from build123d import *

# Parameters (mm, degrees)
SKETCH1_R                   = 79.375
BOSS_EXTRUDE1_DEPTH         = 3.175
TAP_DRILL_FOR_M5X0_8_TAP1_D = 4.2
TAP_DRILL_FOR_M7X1_0_TAP1_D = 6
TAP_DRILL_FOR_M4X0_7_TAP1_D = 3.3


with BuildPart() as part:
    # Sketch1 → Boss-Extrude1 (new, symmetric)
    with BuildSketch(Plane(origin=(0, 0, 0), x_dir=(1, 0, 0), z_dir=(0, 1, 0))):
        with Locations(Location((0, 0, 0), (0, 0, 270))):
            Circle(SKETCH1_R)
    extrude(amount=BOSS_EXTRUDE1_DEPTH, both=True)

    # Tap Drill for M5x0.8 Tap1 (through all)
    with Locations(Plane(origin=(0, 3.175, 0), x_dir=(1, 0, 0), z_dir=(0, 1, 0))):
        with Locations((-27.3188086, 31.571183672), (4.4311914, 31.571183672), (-15.875, -19.245910728), (15.875, -19.245910728)):
            Hole(TAP_DRILL_FOR_M5X0_8_TAP1_D / 2)

    # Tap Drill for M7x1.0 Tap1 (through all)
    with Locations(Plane(origin=(0, 3.175, 0), x_dir=(1, 0, 0), z_dir=(0, 1, 0))):
        with Locations((-44.245, 9.941583672), (-44.245, -15.058416328), (44.245, 9.941583672), (44.245, -15.058416328)):
            Hole(TAP_DRILL_FOR_M7X1_0_TAP1_D / 2)

    # Tap Drill for M4x0.7 Tap1 (through all)
    with Locations(Plane(origin=(0, 3.175, 0), x_dir=(1, 0, 0), z_dir=(0, 1, 0))):
        with Locations((-26.155, -44.384416328), (26.155, -44.384416328)):
            Hole(TAP_DRILL_FOR_M4X0_7_TAP1_D / 2)


solid = part.part
Could you check a few things on this model? Use its own coordinates, in mm. Give positions to 0.01 mm unless a question says otherwise; leave off trailing zeros. Loops run counter-clockwise (first coordinate to the right, second up) from the corner with the lowest first, then second, coordinate; pieces in that order, holes last. Notation, with made-up numbers: M -17,56.5 L 38,56.5 A20 cw 38,94.5 Z; hole C 88,-19.5 d4. An arc over 180 degrees is marked long. Answer as a JSON object with one key per item and string values.
Q1. For P1, Ø1.5, axis at x = 60.5, y = 0.5, coming from the +Z side; P2, Ø2, axis at y = -2, z = -32.5, coming from the +X side; P3, Ø1, axis at x = -23, y = -1, coming from the -Z side, each with a flat end and sliding along its axis, tell me the tip position at first contact or that it passes through.
Values found:
{"P1": "stops at z = 52.25", "P2": "stops at x = 72.86", "P3": "stops at z = -76.12"}
Q2. Suppose I cut it at A-A, the plane y = -0.25. State how many separate pieces and enclosed holes the cut face has, plus the area to 3 significant figures.
Values found:
{"separate pieces": "1", "enclosed holes": "10", "area": "19,600 mm²"}
Q3. If we mould it in two halves opening along Z, with no side actions, what happens to faces 1 (the cylindrical face through (-15.42, -0.044, 21.296)), 2 (the flat face through (1, 3.175, -1)), 3 (the cylindrical face through (23.84, 0.04, 75.71))? For each: pulls with the +Z half, pulls with the -Z half, needs draft (parallel to the pull), parting line crosses it, or undercut.
Values found:
{"face 1": "undercut", "face 2": "needs draft", "face 3": "parting line crosses it"}
Q4. Suppose I cut it at B-B, the plane z = 30. List the corners of the cut face in (x, y) for me (3 decimals).
Values found:
{"outline": "M -73.487,-3.175 L 73.487,-3.175 L 73.487,3.175 L -73.487,3.175 Z"}
Q5. If I drill on probe 1 along X at (y, z) = (-2.5, 21); probe 2 along X at (y, z) = (0.25, -33.5); probe 3 along X at (y, z) = (2.5, 17.5), over which ranges is the centre line in solid material (lowest first)? Write a range as [from, to].
Values found:
{"probe 1": "x = [-76.55, -17.03], [-14.72, 14.72], [17.03, 76.55]", "probe 2": "x = [-71.96, -28.15], [-26.49, 3.6], [5.26, 71.96]", "probe 3": "x = [-77.42, -45.99], [-42.5, -17.04], [-14.71, 14.71], [17.04, 42.5], [45.99, 77.42]"}
Q6. Suppose I cut it at C-C, the plane x = 21. List the corners of the cut face in (y, z) for me (3 decimals), plus the area to 3 significant figures.
Values found:
{"outline": "M -3.175,-76.547 L 3.175,-76.547 L 3.175,76.547 L -3.175,76.547 Z", "area": "972 mm²"}
